Design review of the part built by this model. Coordinates are the model's own, in mm. A direction names the side the tool comes from. Give positions to 0.01 mm unless a question says otherwise; leave off trailing zeros. Loops run counter-clockwise (first coordinate to the right, second up) from the corner with the lowest first, then second, coordinate; pieces in that order, holes last.
from build123d import *

# Parameters (mm, degrees)
F0_R     = 60
F1_DEPTH = 4.9
F3_DEPTH = 4.901
F4_W     = 2
F4_H     = 32
F5_DEPTH = 4.901
F6_W     = 30
F6_H     = 5
F7_DEPTH = 4.901


with BuildPart() as f1:
    # F0 (on Front) → F1 (new body)
    with BuildSketch(Plane.XZ):
        Circle(F0_R)
    extrude(amount=F1_DEPTH)

    # F2 (on face) → F3 (cut, through all)
    with BuildSketch(Plane.XZ.offset(4.9)):
        with BuildLine():
            ThreePointArc((60, 0), (18.3842554453, 57.1140889074), (-48.733971724, 35))
            Line((-48.733971724, 35), (0, 35))
            Line((0, 35), (0, -35))
            Line((0, -35), (-48.733971724, -35))
            ThreePointArc((-48.733971724, -35), (18.3842554453, -57.1140889074), (60, 0))
        make_face()
    extrude(amount=-F3_DEPTH, mode=Mode.SUBTRACT)

    # F4 (on face) → F5 (cut, through all)
    with BuildSketch(Plane.XZ.offset(4.9)):
        with BuildLine():
            Line((-2, -16), (-2, 16))
            ThreePointArc((-2, 16), (-4.4058820349, 0), (-2, -16))
        make_face()
        with Locations((-1, 0)):
            Rectangle(F4_W, F4_H)
    extrude(amount=-F5_DEPTH, mode=Mode.SUBTRACT)

    # F6 (on face) → F7 (cut, through all)
    with BuildSketch(Plane.XZ.offset(4.9)):
        with Locations((-25, 25)):
            Rectangle(F6_W, F6_H)
        with Locations((-25, -25)):
            Rectangle(F6_W, F6_H)
    extrude(amount=-F7_DEPTH, mode=Mode.SUBTRACT)


solid = f1.part
Q1. Take a section at A-A (x = -27). Give the boundary of the cut face in (y, z), plus the area to 3 significant figures.
Results:
outline: (-4.9, -35) - (0, -35) - (0, -27.5) - (-4.9, -27.5) - close; (-4.9, -22.5) - (0, -22.5) - (0, 22.5) - (-4.9, 22.5) - close; (-4.9, 27.5) - (0, 27.5) - (0, 35) - (-4.9, 35) - close
area: 294 mm2
Q2. Take a section at C-C (z = -26.5). Give the boundary of the cut face in (x, y), plus the area to 3 significant figures.
Results:
outline: (-53.83, -4.9) - (-40, -4.9) - (-40, 0) - (-53.83, 0) - close; (-10, -4.9) - (0, -4.9) - (0, 0) - (-10, 0) - close
area: 117 mm2
Q3. Wall thickness on line 1 (Z direction, x = -33.5, y = -0.5); line 2 (X direction, y = -3.9, z = -18); line 3 (X direction, y = -4.45, z = 11): over which ranges is each line inside the solid? List them lowest first.
Results:
line 1: z = -35 to -27.5, -22.5 to 22.5, 27.5 to 35
line 2: x = -57.24 to 0
line 3: x = -58.98 to -3.28
Q4. Insertion check: pin 1 (2 mm diameter, centred on y = -2.5, z = 14, fed in from -X). The pin has a flat end and moves straight along its axis. Give the tip position at first contact, or say it passes through.
Results:
pin 1: stops at x = -58.57
Q5. Tool access review of faces 1 (the face through (-40, -2, -25)), 2 (the face through (-24, -2, -35)), 3 (the face through (-1, -2, -16)): name each direction out of +Z, -Z, +X, -X, +Y, -Y from which nothing blocks a thin tool from reaching the whole face with its end or side.
Results:
face 1: +Y, -Y
face 2: -Z, +X, -X, +Y, -Y
face 3: +X, +Y, -Y
Q6. Take a section at D-D (z = -0.5). Give the boundary of the cut face in (x, y).
Results:
outline: (-60, -4.9) - (-4.4, -4.9) - (-4.4, 0) - (-60, 0) - close
Q7. Take a section at B-B (y = -1.6). Give the boundary of the cut face in (x, z), plus the area to 3 significant figures.
Results:
outline: (-48.73, -35) - (0, -35) - (0, -16) - (-2, -16) arc R54.41 cw to (-2, 16) - (0, 16) - (0, 35) - (-48.73, 35) arc R60 ccw to start; hole (-40, -27.5) - (-10, -27.5) - (-10, -22.5) - (-40, -22.5) - close; hole (-40, 22.5) - (-10, 22.5) - (-10, 27.5) - (-40, 27.5) - close
area: 3,530 mm2
Q8. Draft analysis for pull direction X (two halves, no side actions). For faces 4 (the face through (-10, -2, -25)), 5 (the face through (-25, -2, 35)), 6 (the face through (-25, -2, 27.5)), 7 (the face through (0, -2, -25)), state which applies: pulls with the +X half, pulls with the -X half, needs draft (parallel to the pull), parting line crosses it, or undercut.
Results:
face 4: undercut
face 5: needs draft
face 6: undercut
face 7: pulls with the +X half
